For this review, take the finished solid that the model builds, in its own axes (mm). Coordinates: 2 decimals unless noted, no trailing zeros. Order: outer loops, then holes, each group sorted by start corner. A loop starts at its lowest first (then second) coordinate and runs counter-clockwise, first axis right, second up. Notation, with made-up numbers: (-32, 36) -> (3, 36) arc R31 ccw to (3, 72) -> close; hole circle Ø9 at (-34, 80). An arc over 180 degrees is marked (long way). Write item = value, one per line. Start each with the question number.
1) Wall thickness on probe 1 along Z at (x, y) = (-1.25, 6.5); probe 2 along Y at (x, z) = (0, 4); probe 3 along X at (y, z) = (23, 3.5): over which ranges is each line inside the solid? List them lowest first. Write a range as [from, to].
2) Consider section A-A on y = 13. Give the boundary of the cut face in (x, z), and give its area (3 significant figures).
3) Consider section B-B on x = 0. Give the boundary of the cut face in (y, z), and give its area (3 significant figures).
4) Insertion check: pin 1 Ø1.9 at (y, z) = (7, 3.5) entering from -X; pin 2 Ø0.6 at (y, z) = (-9.5, 0.5) entering from -X; pin 3 Ø0.9 at (y, z) = (-2, 0.5) entering from +X. Each pin has a flat end and moves straight along its axis. Give the tip position at first contact, or say it passes through.
5) Consider section C-C on z = 2. Give the boundary of the cut face in (x, y).
6) Consider section D-D on x = -3.5. Give the boundary of the cut face in (y, z), and give its area (3 significant figures).
from build123d import *

# Parameters (mm, degrees)
SKETCH1_W             = 4
SKETCH1_H             = 66
BOSS_EXTRUDE1_DEPTH   = 1
SKETCH1_2_W           = 4
SKETCH1_2_H           = 66
BOSS_EXTRUDE2_DEPTH   = 1.36844839
SKETCH4_W             = 2
SKETCH4_H             = 66.494663906
BOSS_EXTRUDE3_DEPTH   = 5
SKETCH4_2_W           = 2
SKETCH4_2_H           = 66.494663906
BOSS_EXTRUDE4_DEPTH   = 6.842238407
F_3_0MM_DOWEL_HOLE1_D = 3
SKETCH9_W             = 9
SKETCH9_H             = 72.967983433
BOSS_EXTRUDE6_DEPTH   = 4


with BuildPart() as part:
    # Sketch1 → Boss-Extrude1 (new, along a direction that is not the sketch's normal)
    with BuildSketch(Plane.XY):
        Rectangle(SKETCH1_W, SKETCH1_H)
    extrude(amount=BOSS_EXTRUDE1_DEPTH, dir=(0, 0.6347305132022716, 0.7727335734973478))

    # Sketch1<2> → Boss-Extrude2 (add, along a direction that is not the sketch's normal)
    with BuildSketch(Plane.XY):
        Rectangle(SKETCH1_2_W, SKETCH1_2_H)
    extrude(amount=BOSS_EXTRUDE2_DEPTH, dir=(0, 0.8253106586930028, 0.5646789500660725))

    # Sketch4 → Boss-Extrude3 (add, along a direction that is not the sketch's normal)
    with BuildSketch(Plane.XY.offset(0.772733573)):
        with Locations((0, 0.882062466)):
            Rectangle(SKETCH4_W, SKETCH4_H)
    extrude(amount=BOSS_EXTRUDE3_DEPTH, dir=(0, 0.6347305132022716, 0.7727335734973478))

    # Sketch4<2> → Boss-Extrude4 (add, along a direction that is not the sketch's normal)
    with BuildSketch(Plane.XY.offset(0.772733573)):
        with Locations((0, 0.882062466)):
            Rectangle(SKETCH4_2_W, SKETCH4_2_H)
    extrude(amount=BOSS_EXTRUDE4_DEPTH, dir=(0, 0.8253106586930028, 0.5646789500660725))

    # Ø3.0mm Dowel Hole1 (through all)
    with Locations(Plane.ZY.offset(1)):
        with Locations((2.704567507, -14.191616921), (2.704567507, 15.808383079)):
            Hole(F_3_0MM_DOWEL_HOLE1_D / 2)

    # Sketch9 → Boss-Extrude6 (add)
    with BuildSketch(Plane.XY.offset(4.636401441)):
        with Locations((0, 3.292374795)):
            Rectangle(SKETCH9_W, SKETCH9_H)
    extrude(amount=BOSS_EXTRUDE6_DEPTH)


solid = part.part
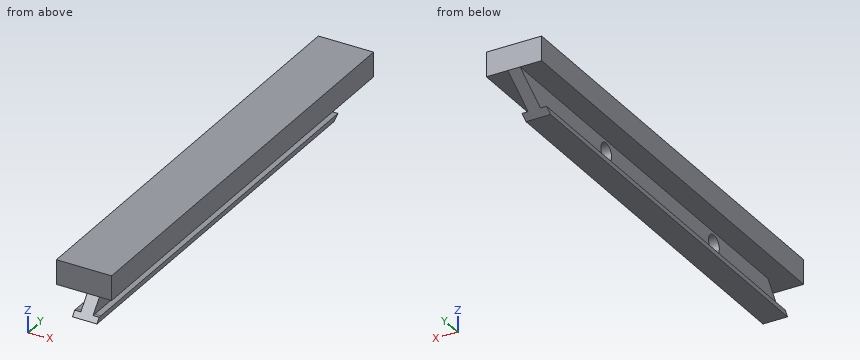
Answer sheet:
q1.probe_1 = [0, 0.77], [4.64, 8.64]
q1.probe_2 = [-29.71, -14.95], [-13.44, 15.05], [16.56, 38.85]
q1.probe_3 = [-1, 1]
q2.outline = (-4.5, 4.64) -> (-1, 4.64) -> (-1, 0.77) -> (-2, 0.77) -> (-2, 0) -> (2, 0) -> (2, 0.77) -> (1, 0.77) -> (1, 4.64) -> (4.5, 4.64) -> (4.5, 8.64) -> (-4.5, 8.64) -> close
q2.area = 46.8 mm2
q3.outline = (-33.19, 4.64) -> (-29.19, 4.64) -> (-33, 0) -> (33, 0) -> (39.78, 4.64) -> (39.78, 8.64) -> (-33.19, 8.64) -> close; hole circle Ø3 at (-14.19, 2.7); hole circle Ø3 at (15.81, 2.7)
q3.area = 591 mm2
q4.pin_1 = -1
q4.pin_2 = -2
q4.pin_3 = 2
q5.outline = (-1, -31.36) -> (1, -31.36) -> (1, -15.52) -> (-1, -15.52) -> close; (-1, -12.87) -> (1, -12.87) -> (1, 14.48) -> (-1, 14.48) -> close; (-1, 17.13) -> (1, 17.13) -> (1, 35.92) -> (-1, 35.92) -> close
q6.outline = (-33.19, 4.64) -> (39.78, 4.64) -> (39.78, 8.64) -> (-33.19, 8.64) -> close
q6.area = 292 mm2
